Source: CAD feature listing. Evaluate the final solid. Frame: model axes, mm. A direction names the side the tool comes from. Give positions to 0.01 mm unless a question says otherwise; leave off trailing zeros. Write each loop counter-clockwise with the first axis right and the second up, starting at its lowest first coordinate (ties: lowest second). Pieces come first, ordered by that corner, then holes. Notation, with made-up numbers: (-20, 77.25) -> (20, 77.25) arc R28 ccw to (20, 109.25) -> close; hole circle Ø6 at (-35.5, 82). An arc over 180 degrees is marked (long way). Write item = value, one per line.
from build123d import *

# Parameters (mm, degrees)
SKETCH1_W           = 41
SKETCH1_H           = 41
BOSS_EXTRUDE1_DEPTH = 6
SKETCH2_R           = 1.5
CUT_EXTRUDE1_DEPTH  = 6
SKETCH3_W           = 26
SKETCH3_H           = 26
CUT_EXTRUDE2_DEPTH  = 6
FILLET1_R           = 3


with BuildPart() as part:
    # Sketch1 → Boss-Extrude1 (new body)
    with BuildSketch(Plane(origin=(0, 0, 0), x_dir=(1, 0, 0), z_dir=(0, 1, 0))):
        Rectangle(SKETCH1_W, SKETCH1_H)
    extrude(amount=BOSS_EXTRUDE1_DEPTH)

    # Sketch2 → Cut-Extrude1 (cut)
    with BuildSketch(Plane(origin=(0, 0, 0), x_dir=(1, 0, 0), z_dir=(0, 1, 0))):
        with Locations((-15.5, 15.5)):
            Circle(SKETCH2_R)
        with Locations((15.5, 15.5)):
            Circle(SKETCH2_R)
        with Locations((-15.5, -15.5)):
            Circle(SKETCH2_R)
        with Locations((15.5, -15.5)):
            Circle(SKETCH2_R)
    extrude(amount=CUT_EXTRUDE1_DEPTH, mode=Mode.SUBTRACT)

    # Sketch3 → Cut-Extrude2 (cut)
    with BuildSketch(Plane(origin=(0, 0, 0), x_dir=(1, 0, 0), z_dir=(0, 1, 0))):
        Rectangle(SKETCH3_W, SKETCH3_H)
    extrude(amount=CUT_EXTRUDE2_DEPTH, mode=Mode.SUBTRACT)

    # Fillet1
    fillet1_edges = [part.edges().sort_by_distance(p)[0] for p in [
        (13, 3, 13),
        (13, 3, -13),
        (-13, 3, -13),
        (-13, 3, 13),
        (20.5, 3, 20.5),
        (-20.5, 3, 20.5),
        (-20.5, 3, -20.5),
        (20.5, 3, -20.5),
    ]]
    fillet(fillet1_edges, radius=FILLET1_R)


solid = part.part
1) Cut plane B-B (z = 1). Return the cut outline in (x, y), then the cut area to 3 significant figures.
Computed:
outline = (-20.5, 0) -> (-13, 0) -> (-13, 6) -> (-20.5, 6) -> close; (13, 0) -> (20.5, 0) -> (20.5, 6) -> (13, 6) -> close
area = 90.0 mm²
2) Draft query along Z for faces 1 (the cylindrical face through (19.6, 3.04, -19.64)), 2 (the cylindrical face through (-19.64, 3.04, 19.6)), 3 (the flat face through (0, 3, 13)). Return one class per face: pulls with the +Z half, pulls with the -Z half, needs draft (parallel to the pull), parting line crosses it, or undercut.
Computed:
face_1 = pulls with the -Z half
face_2 = pulls with the +Z half
face_3 = undercut
3) Cut plane C-C (y = 2.9). Return the cut outline in (x, z).
Computed:
outline = (-20.5, -17.5) arc R3 ccw to (-17.5, -20.5) -> (17.5, -20.5) arc R3 ccw to (20.5, -17.5) -> (20.5, 17.5) arc R3 ccw to (17.5, 20.5) -> (-17.5, 20.5) arc R3 ccw to (-20.5, 17.5) -> close; hole circle Ø3 at (-15.5, -15.5); hole circle Ø3 at (-15.5, 15.5); hole (-13, -10) arc R3 ccw to (-10, -13) -> (10, -13) arc R3 ccw to (13, -10) -> (13, 10) arc R3 ccw to (10, 13) -> (-10, 13) arc R3 ccw to (-13, 10) -> close; hole circle Ø3 at (15.5, -15.5); hole circle Ø3 at (15.5, 15.5)
4) Cut plane D-D (z = -15.5). Return the cut outline in (x, y).
Computed:
outline = (-20.5, 0) -> (-17, 0) -> (-17, 6) -> (-20.5, 6) -> close; (-14, 0) -> (14, 0) -> (14, 6) -> (-14, 6) -> close; (17, 0) -> (20.5, 0) -> (20.5, 6) -> (17, 6) -> close
5) Cut plane A-A (x = 15.5). Return the cut outline in (y, z).
Computed:
outline = (0, -20.5) -> (6, -20.5) -> (6, -17) -> (0, -17) -> close; (0, -14) -> (6, -14) -> (6, 14) -> (0, 14) -> close; (0, 17) -> (6, 17) -> (6, 20.5) -> (0, 20.5) -> close
6) Access query for faces 4 (the flat face through (13, 3, 0)), 5 (the cylindrical face through (19.6, 3.04, 19.64)). Directions: +Z, -Z, +X, -X, +Y, -Y. A direction counts if a zero-diameter tool reaches every point of the face in a straight line with its end or side. Return the directions, or none.
Computed:
face_4 = +Y, -Y
face_5 = +Z, +X, +Y, -Y
7) Material intervals for L1, parallel to X at y = 3.2, z = 15.5; L2, parallel to Z at x = -2, y = 4.25, sorted ascending.
Computed:
L1 = -20.5 to -17, -14 to 14, 17 to 20.5
L2 = -20.5 to -13, 13 to 20.5
